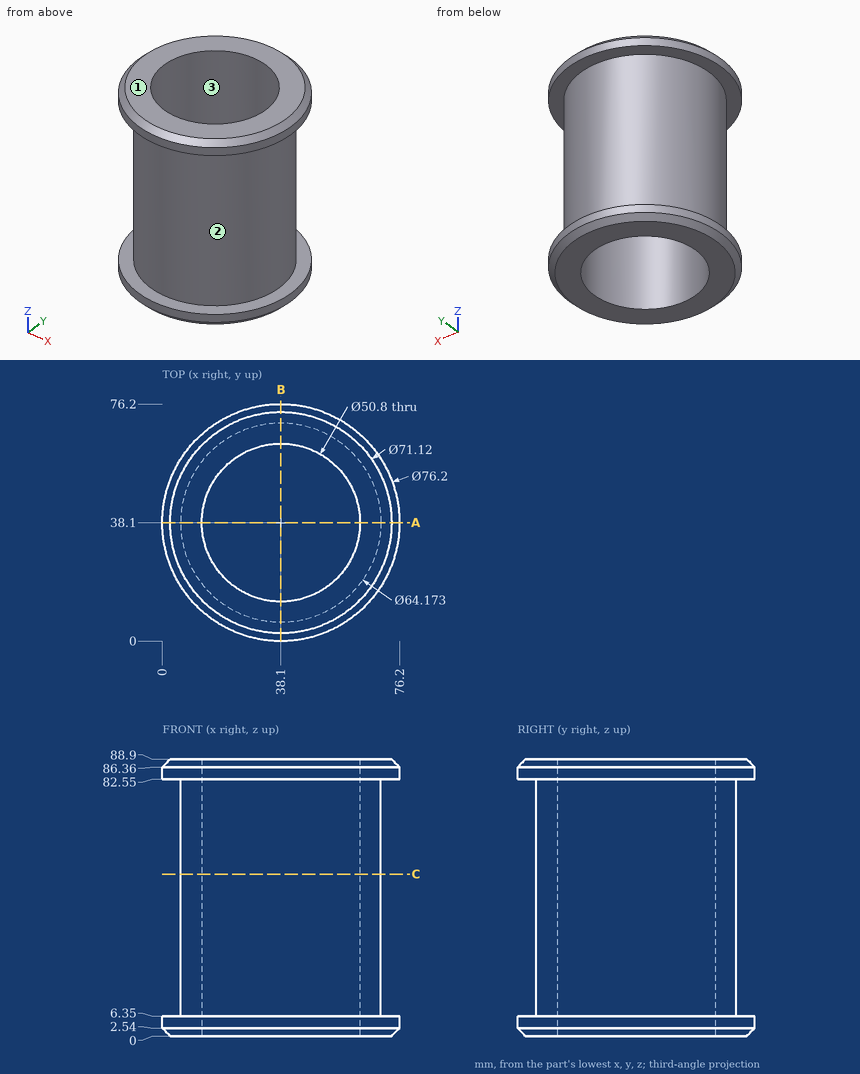
For this review, use the dimensioned drawing (mm, ordinates from the lowest corner) and the shaded views. Coordinates: 2 decimals unless noted, no trailing zeros. Order: outer loops, then holes, each group sorted by start corner. A loop starts at its lowest first (then second) coordinate and runs counter-clockwise, first axis right, second up. Notation, with made-up numbers: M 24,-2 L 72,-2 A26 ccw 72,23 Z; hole C 26,62.25 d8. An arc over 180 degrees is marked long. Answer as a JSON object with one key per item and string values. Group by question number.
1) Add section A-A, the plane y = 38.1. Write out the cut boundary in (x, z).
2) Wall thickness on L1, parallel to Y at x = 38, z = 45; L2, parallel to Y at x = 30.5, z = 31: over which ranges is each line inside the solid? List them lowest first.
3) Add section C-C, the plane z = 52. Write out the cut boundary in (x, y).
4) For pin 1 (1 mm diameter, centred on x = 47, z = 18.5, fed in from +Y); pin 2 (3 mm diameter, centred on x = 29, z = 11, fed in from +Y); pin 3 (23 mm diameter, centred on x = 42.5, y = 49, fed in from -Z); pin 4 (8 mm diameter, centred on y = 43.5, z = 50.5, fed in from -X), all flat-tipped, find the tip position at first contact; note any pin that passes through.
5) Mouldability with a two-part tool opening along X and no side actions: class the marked faces 1, 2 and 3 as pulls with the +X half, pulls with the -X half, needs draft (parallel to the pull), parting line crosses it, or undercut.
Computed values:
{
 "1": {"outline": "M 0,2.54 L 2.54,0 L 12.7,0 L 12.7,88.9 L 2.54,88.9 L 0,86.36 L 0,82.55 L 6.01,82.55 L 6.01,6.35 L 0,6.35 Z; M 63.5,0 L 73.66,0 L 76.2,2.54 L 76.2,6.35 L 70.19,6.35 L 70.19,82.55 L 76.2,82.55 L 76.2,86.36 L 73.66,88.9 L 63.5,88.9 Z"},
 "2": {"L1": "y = 6.01 to 12.7, 63.5 to 70.19", "L2": "y = 6.93 to 13.86, 62.34 to 69.27"},
 "3": {"outline": "C 38.1,38.1 d64.17; hole C 38.1,38.1 d50.8"},
 "4": {"pin 1": "stops at y = 69.07", "pin 2": "stops at y = 69.27", "pin 3": "passes through", "pin 4": "stops at x = 6.04"},
 "5": {"face 1": "needs draft", "face 2": "parting line crosses it", "face 3": "undercut"}
}
